from build123d import *

# Parameters (mm, degrees)
EXTRUDE_1_DEPTH = 5
FILLET_1_R      = 0.5


with BuildPart() as part:
    # Эскиз1 → Бобышка-Вытянуть1 (new body)
    with BuildSketch(Plane.XY):
        with BuildLine():
            Line((0.352984217, 0), (0, 0))
            ThreePointArc((0, 0), (-1.379289319, 0.551704113), (-1.997619047, 1.902439024))
            ThreePointArc((-1.997619047, 1.902439024), (9.812828894, 33.65472035), (40.951190459, 47))
            Line((40.951190459, 47), (57.951190459, 47))
            ThreePointArc((57.951190459, 47), (60.072510802, 46.121320344), (60.951190459, 44))
            Line((60.951190459, 44), (60.951190459, 42))
            ThreePointArc((60.951190459, 42), (60.072510802, 39.878679656), (57.951190459, 39))
            Line((57.951190459, 39), (44.951190459, 39))
            ThreePointArc((44.951190459, 39), (16.645125149, 28.369224066), (2.335126717, 1.733333333))
            ThreePointArc((2.335126717, 1.733333333), (1.669545394, 0.494454695), (0.352984217, 0))
        make_face()
    extrude(amount=EXTRUDE_1_DEPTH)

    # Скругление1
    fillet_1_edges = [part.edges().sort_by_distance(p)[0] for p in [
        (51.451190459, 39, 5),
        (60.072510802, 39.878679656, 5),
        (60.951190459, 43, 5),
        (60.072510802, 46.121320344, 5),
        (49.451190459, 47, 5),
        (9.812828894, 33.65472035, 5),
        (-1.379289319, 0.551704113, 5),
        (0.176492108, 0, 5),
        (1.669545394, 0.494454695, 5),
        (16.645125149, 28.369224066, 5),
    ]]
    fillet(fillet_1_edges, radius=FILLET_1_R)


solid = part.part
Geometry check sheet. Reference: the model listing, model coordinates, mm. A direction names the side the tool comes from. Round coordinates to 2 decimals unless told otherwise and drop trailing zeros. Write each loop counter-clockwise with the first axis right and the second up, starting at its lowest first coordinate (ties: lowest second). Pieces come first, ordered by that corner, then holes.
Item 1: Access from +Z, -Z, +X, -X, +Y, -Y to the whole of each face (thin tool, end or side, straight path). Record for faces 1 (the face through (60.951, 43, 2)), 2 (the face through (52, 39, 2)).
Determined:
face 1: +Z, -Z, +X, +Y, -Y
face 2: +Z, -Z, +X, -Y
Item 2: Go/stop test with a flat-tipped pin: pin 1 Ø6 at (x, y) = (5, 34) entering from -Z. Record where the tip stops, or that it passes through.
Determined:
pin 1: passes through
Item 3: Material ranges on line 1 along Z through (x, y) = (28, 36); line 2 along Y through (x, z) = (55, 4); line 3 along X through (y, z) = (9, 1.3), recorded low to high.
Determined:
line 1: z = 0 to 5
line 2: y = 39 to 47
line 3: x = -1.76 to 3.96
Item 4: Section check B-B (x = 51). Record the boundary of the cut face in (y, z), plus the area to 3 significant figures.
Determined:
outline: (39, 0) - (47, 0) - (47, 4.5) arc R0.5 ccw to (46.5, 5) - (39.5, 5) arc R0.5 ccw to (39, 4.5) - close
area: 39.9 mm2
Item 5: Section check A-A (z = 2.7). Record the boundary of the cut face in (x, y), plus the area to 3 significant figures.
Determined:
outline: (-2, 1.9) arc R2 ccw to (0, 0) - (0.35, 0) arc R2 ccw to (2.34, 1.73) arc R43 cw to (44.95, 39) - (57.95, 39) arc R3 ccw to (60.95, 42) - (60.95, 44) arc R3 ccw to (57.95, 47) - (40.95, 47) arc R43 ccw to start
area: 654 mm2
